Autodesk Inventor part; units mm, degrees
ref_plane "YZ Plane" through (0, 0, 0) normal (1, 0, 0) x (0, 1, 0)
ref_plane "XZ Plane" through (0, 0, 0) normal (0, 1, 0) x (-1, 0, 0)
ref_plane "XY Plane" through (0, 0, 0) normal (0, 0, 1) x (1, 0, 0)
sketch "Sketch2" plane through (0, 0, 0) normal (0, 1, 0) x (-1, 0, 0)
  line L0 (101.6465, 0) -> (-102.4493, 0)
  line L1 (0, -49.7697) -> (0, 40.9396)
  line L2 (0, -27.5) -> (80, -27.5)
  line L3 (88, -27.5) -> (88, -25) construction
  line L4 (84, -25) -> (82, -25)
  line L5 (80.5, -26.5) -> (80.5, -27)
  line L6 (88, -21) -> (88, 0)
  line L7 (80.5, -27.5) -> (88, -27.5) construction
  arc A0 (84, -25) -> (88, -21) centre (84, -21) ccw
  arc A1 (82, -25) -> (80.5, -26.5) centre (82, -26.5) ccw
  arc A2 (80, -27.5) -> (80.5, -27) centre (80, -27) ccw
  circle A3 centre (84, -21) radius 1.6
  point P0 (0, 0)
  dimension "d7" = 176
  dimension "d8" = 55
  dimension "d9" = 2.5
  dimension "d10" = 7.5
  dimension "d11" = 4
  dimension "d12" = 1.5
  dimension "d13" = 0.5
  dimension "d16" = 3.2
extrude "Extrusion1" add sketch "Sketch2" along normal blind 1.6
mirror "Mirror1" about plane through (0, 0, 0) normal (0, 0, 1) of "Extrusion1"
mirror "Mirror2" about plane through (0, 0, 0) normal (1, 0, 0) of "Extrusion1", "Mirror1"
sketch "Sketch3" plane through (0, 1.6, 0) normal (0, 1, 0) x (1, 0, 0)
  line L0 (-54.5, 30) -> (-45.5, 30)
  line L1 (-45.5, 30) -> (-45.5, 15.2)
  line L2 (-45.5, 15.2) -> (-54.5, 15.2)
  line L3 (-54.5, 15.2) -> (-54.5, 30)
  point P0 (0, 0)
  point P1 (-50, 25)
  point P2 (-50, 30)
  dimension "d17" = 50
  dimension "d18" = 25
  dimension "d19" = 9
  dimension "d20" = 14.8
  dimension "d21" = 5
extrude "Extrusion2" add sketch "Sketch3" along normal blind 11
sketch "Sketch4" plane through (-45.5, 1.6, -30) normal (0, 0, -1) x (-1, 0, 0)
  circle A0 centre (4.5, 6.5) radius 3.25
  line L0 (0, 11) -> (9, 11)
  line L1 (9, 0) -> (0, 0)
  circle A1 centre (4.5, 6.5) radius 1
  point P0 (-45.5, -1.6)
  point P1 (4.5, 11)
  point P2 (4.5, 11)
  dimension "d24" = 6.5
  dimension "d25" = 6.5
  dimension "d26" = 2
extrude "Extrusion3" cut sketch "Sketch4" against normal blind 11
sketch "Sketch5" plane through (0, 1.6, 0) normal (0, 1, 0) x (1, 0, 0)
  line L0 (56, 19.4) -> (49, 19.4)
  line L1 (49, 19.4) -> (49, 26.4)
  line L2 (49, 26.4) -> (56, 26.4)
  line L3 (56, 26.4) -> (56, 19.4)
  line L4 (56, 19.4) -> (49, 26.4) construction
  line L5 (49, 19.4) -> (56, 26.4) construction
  point P0 (0, 0)
  point P1 (52.5, 22.9)
  dimension "d29" = 52.5
  dimension "d30" = 22.9
  dimension "d31" = 7
extrude "Extrusion4" add sketch "Sketch5" along normal blind 10
sketch "Sketch6" plane through (56, 1.6, -26.4) normal (0, 0, -1) x (-1, 0, 0)
  line L0 (0, 10) -> (7, 10)
  circle A0 centre (3.5, 6.6) radius 3.4
  line L1 (101.5, 0) -> (-24, 0)
  point P0 (56, -1.6)
  point P1 (3.5, 10)
  dimension "d34" = 6.6
  dimension "d35" = 6.8
extrude "Extrusion5" add sketch "Sketch6" along normal blind 1.1
sketch "Sketch7" plane through (52.5, 8.2, -27.5) normal (0, 0, -1) x (-1, 0, 0)
  circle A0 centre (0, 0) radius 3.4
  circle A1 centre (0, 0) radius 3.175
  point P0 (52.5, -8.2)
  dimension "d38" = 6.35
extrude "Extrusion6" add sketch "Sketch7" along normal blind 11.4 contours A1
sketch "Sketch8" plane through (0, 1.6, 0) normal (0, 1, 0) x (1, 0, 0)
  line L0 (23.75, 28.02) -> (31.25, 28.02)
  line L1 (31.25, 28.02) -> (31.25, 22.45)
  line L2 (31.25, 22.45) -> (23.75, 22.45)
  line L3 (23.75, 22.45) -> (23.75, 28.02)
  point P0 (0, 0)
  point P1 (27.5, 27.5)
  point P2 (27.5, 28.02)
  dimension "d41" = 27.5
  dimension "d42" = 27.5
  dimension "d43" = 5.05
  dimension "d44" = 0.52
  dimension "d45" = 7.5
extrude "Extrusion7" add sketch "Sketch8" along normal blind 2.7
equation "\"BendRadius\" = Thickness"
equation "\"BendReliefWidth\" = Thickness"
equation "\"BendReliefDepth\" = 0.5 * Thickness"
equation "\"CornerReliefSize\" = 4 * Thickness"
equation "\"MinimumRemnant\" = 2 * Thickness"
equation "\"TransitionRadius\" = BendRadius"
equation "\"JacobiRadiusSize\" = BendRadius"
equation "\"GapSize\" = Thickness"
properties part number "MainPCB"
Here's how the part is built. I have some questions about the finished solid (model axes, mm). A direction names the side the tool comes from. Round coordinates to 2 decimals unless told otherwise and drop trailing zeros. Loops run counter-clockwise (first coordinate to the right, second up) from the corner with the lowest first, then second, coordinate; pieces in that order, holes last. Notation, with made-up numbers: M 75.25,26 L 116.25,26 A27 cw 116.25,58 Z; hole C 5,17 d10. An arc over 180 degrees is marked long. Write each question's results on one line, items separated by ' | '. Start each with the question number.
(1) Will these pins go through, and if not, where does the flat tip stop? P1, Ø4, axis at x = -0.5, y = 4.5, coming from the -Z side; P2, Ø10, axis at x = -19, z = -17.5, coming from the +Y side; P3, Ø1.6, axis at x = -50, y = 8.5, coming from the -Z side; P4, Ø2, axis at y = 3.5, z = -25, coming from the -X side.
(2) On a 3-axis mill with a long thin cutter (end or side, diameter ignored), from which of +Z, -Z, +X, -X, +Y, -Y can I reach the whole of each face in a straight line? I mean faces 1 (the flat face through (52, 4, -26.4)), 2 (the flat face through (49, 7, -23)), 3 (the flat face through (-54.5, 7, -22)). Say none if no direction works.
(3) I want a section at A-A (x = -11). Please give me the cut outline in (y, z), then the cut area to 3 significant figures.
(4) Thinking about a two-plate mould opening in X: for faces 4 (the flat face through (56, 7, -23)), 5 (the flat face through (52, 11.6, -23)), 6 (the cylindrical face through (-82.4, 0.79, -21.07)), which applies, pulls with the +X half, pulls with the -X half, needs draft (parallel to the pull), parting line crosses it, or undercut?
(5) If I drill on probe 1 along Z at (x, y) = (84, 1.2); probe 2 along X at (y, z) = (0.4, 21); probe 3 along Y at (x, z) = (48.5, -10.5), over which ranges is the centre line in solid material (lowest first)? Write a range as from..to.
Solved:
1) P1: passes through | P2: stops at y = 1.6 | P3: stops at z = -30 | P4: stops at x = -54.5
2) face 1: -Z | face 2: +Z, -Z, +Y | face 3: +Z, -Z, -X, +Y
3) outline: M 0,-27.5 L 1.6,-27.5 L 1.6,27.5 L 0,27.5 Z | area: 88.0 mm²
4) face 4: pulls with the +X half | face 5: needs draft | face 6: undercut
5) probe 1: z = -25..-22.6, -19.4..19.4, 22.6..25 | probe 2: x = -88..-85.6, -82.4..82.4, 85.6..88 | probe 3: y = 0..1.6
